Geometry check sheet. Reference: the model listing, model coordinates, mm. Face numbers are marked on the shaded views. A direction names the side the tool comes from. Give positions to 0.01 mm unless a question says otherwise; leave off trailing zeros. Order: outer loops, then holes, each group sorted by start corner. A loop starts at its lowest first (then second) coordinate and runs counter-clockwise, first axis right, second up. Notation, with made-up numbers: M 1.25,31.5 L 58.25,31.5 A19 cw 58.25,61.5 Z; hole C -14.75,49 d1. An arc over 180 degrees is marked long. Answer as CSV lines item,"result". Start each with the question number.
```python
from build123d import *

# Parameters (mm, degrees)
BOSS_EXTRUDE1_DEPTH = 10
BOSS_EXTRUDE2_START = 1
BOSS_EXTRUDE2_DEPTH = 1
SKETCH3_R           = 4
BOSS_EXTRUDE3_DEPTH = 6
SKETCH4_R           = 2
BOSS_EXTRUDE4_DEPTH = 15
FILLET1_R           = 2


with BuildPart() as part:
    # Sketch1 → Boss-Extrude1 (new body)
    with BuildSketch(Plane(origin=(0, 0, 0), x_dir=(1, 0, 0), z_dir=(0, 1, 0))):
        with BuildLine():
            Line((-20.000157194, 1.500878546), (-20.000157194, -1.500878546))
            Line((-20.000157194, -1.500878546), (-0.880639137, -4.921836518))
            ThreePointArc((-0.880639137, -4.921836518), (0, -5), (0.880639137, -4.921836518))
            Line((0.880639137, -4.921836518), (20.000157194, -1.500878546))
            Line((20.000157194, -1.500878546), (20.000157194, 1.500878546))
            Line((20.000157194, 1.500878546), (0.880639137, 4.921836518))
            ThreePointArc((0.880639137, 4.921836518), (0, 5), (-0.880639137, 4.921836518))
            Line((-0.880639137, 4.921836518), (-20.000157194, 1.500878546))
        make_face()
        with BuildLine():
            Line((-19.000157194, -0.663922493), (-19.000157194, 0.663922493))
            Line((-19.000157194, 0.663922493), (-18.824029366, 0.695436148))
            Line((-18.824029366, 0.695436148), (-3.65761322, 3.409085733))
            ThreePointArc((-3.65761322, 3.409085733), (-5, 0), (-3.65761322, -3.409085733))
            Line((-3.65761322, -3.409085733), (-18.824029366, -0.695436148))
            Line((-18.824029366, -0.695436148), (-19.000157194, -0.663922493))
        make_face(mode=Mode.SUBTRACT)
        with BuildLine():
            Line((18.824029366, 0.695436148), (19.000157194, 0.663922493))
            Line((19.000157194, 0.663922493), (19.000157194, -0.663922493))
            Line((19.000157194, -0.663922493), (18.824029366, -0.695436148))
            Line((18.824029366, -0.695436148), (3.65761322, -3.409085733))
            ThreePointArc((3.65761322, -3.409085733), (5, 0), (3.65761322, 3.409085733))
            Line((3.65761322, 3.409085733), (18.824029366, 0.695436148))
        make_face(mode=Mode.SUBTRACT)
    extrude(amount=BOSS_EXTRUDE1_DEPTH)

    # Sketch2 → Boss-Extrude2 (add)
    with BuildSketch(Plane.XZ.offset(BOSS_EXTRUDE2_START)):
        with BuildLine():
            Line((-20.000157194, 1.500878546), (-0.880639137, 4.921836518))
            ThreePointArc((-0.880639137, 4.921836518), (0, 5), (0.880639137, 4.921836518))
            Line((0.880639137, 4.921836518), (20.000157194, 1.500878546))
            Line((20.000157194, 1.500878546), (20.000157194, -1.500878546))
            Line((20.000157194, -1.500878546), (0.880639137, -4.921836518))
            ThreePointArc((0.880639137, -4.921836518), (0, -5), (-0.880639137, -4.921836518))
            Line((-0.880639137, -4.921836518), (-20.000157194, -1.500878546))
            Line((-20.000157194, -1.500878546), (-20.000157194, 1.500878546))
        make_face()
    extrude(amount=-BOSS_EXTRUDE2_DEPTH)

    # Sketch3 → Boss-Extrude3 (add)
    with BuildSketch(Plane(origin=(0, 10, 0), x_dir=(1, 0, 0), z_dir=(0, 1, 0))):
        with Locations(Location((0, 0, 0), (0, 0, 270))):
            Circle(SKETCH3_R)
    extrude(amount=BOSS_EXTRUDE3_DEPTH)

    # Sketch4 → Boss-Extrude4 (add)
    with BuildSketch(Plane(origin=(0, 16, 0), x_dir=(1, 0, 0), z_dir=(0, 1, 0))):
        with Locations(Location((0, 0, 0), (0, 0, 270))):
            Circle(SKETCH4_R)
    extrude(amount=BOSS_EXTRUDE4_DEPTH)

    # Fillet1
    # the kernel refuses this fillet: 2 mm, written as the material it takes off along each edge
    with BuildSketch(Plane(origin=(20.000157194, -5.184780263, 1.500878546), x_dir=(-0.9843673036221247, 0, 0.17612782732920945), z_dir=(0, 1, 0)), Plane(origin=(20.000157194, -5.184780263, -1.500878546), x_dir=(0, 0, 1), z_dir=(0, 1, 0)), Plane(origin=(-20.000157194, 14.184780263, 1.500878546), x_dir=(0.9843673036221245, 0, 0.17612782732920956), z_dir=(0, -1, 0))) as fillet1_piece_1:
        with BuildLine():
            CenterArc((FILLET1_R * 0.836956052521, -FILLET1_R), FILLET1_R, 90, 79.855702636)
            Line((-FILLET1_R * 0.147411251101, -FILLET1_R * 0.823872172671), (0, 0))
            Line((0, 0), (FILLET1_R * 0.836956052521, 0))
        make_face()
    extrude(amount=19.369560525, mode=Mode.SUBTRACT)
    with BuildSketch(Plane(origin=(-20.000157194, -5.184780263, -1.500878546), x_dir=(0, 0, 1), z_dir=(0, 1, 0))) as fillet1_piece_2:
        with BuildLine():
            CenterArc((FILLET1_R * 0.836956052521, FILLET1_R), FILLET1_R, 190.144297364, 79.855702636)
            Line((-FILLET1_R * 0.147411251101, FILLET1_R * 0.823872172671), (0, 0))
            Line((0, 0), (FILLET1_R * 0.836956052521, 0))
        make_face()
    extrude(amount=19.369560525, mode=Mode.SUBTRACT)


solid = part.part
```
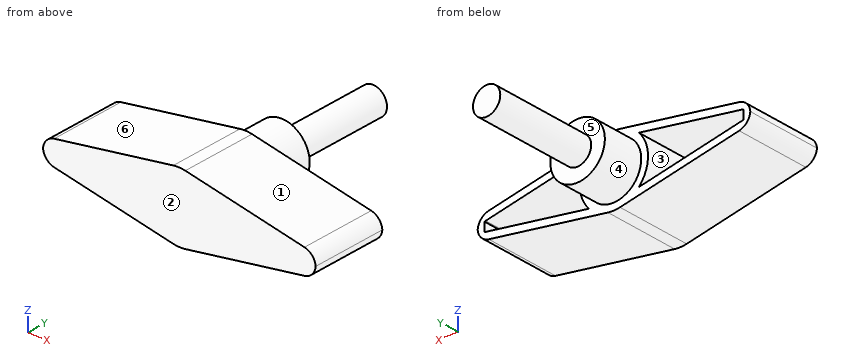
Item 1: Section check D-D on x = -8. Record the boundary of the cut face in (y, z).
Item 2: Draft check along X on the marked faces 1, 2, 3 and 4. Enter one of: pulls with the +X half, pulls with the -X half, needs draft (parallel to the pull), parting line crosses it, or undercut.
Item 3: Access from +Z, -Z, +X, -X, +Y, -Y to the whole of each face (thin tool, end or side, straight path). Record for the marked faces 5 and 6.
Item 4: Depth check by flat-ended pin: pin 1 Ø2 at (x, z) = (10, 0) entering from +Y; pin 2 Ø5.5 at (x, z) = (-11, 1.5) entering from +Y; pin 3 Ø6 at (x, y) = (-4, 3.5) entering from +Z. Enter the tip coordinate at first touch or a pass-through.
Item 5: Section check B-B on y = 18.5. Record the boundary of the cut face in (x, z).
Item 6: Scan lines: line 1 along Y through (x, z) = (3.5, -2.5); line 2 along Z through (x, y) = (-14, 2); line 3 along Y through (x, z) = (6, -1.75). Record each from-to range of solid material in increasing order.
Item 7: Section check C-C on z = -2.5. Record the boundary of the cut face in (x, y), then the cut area to 3 significant figures.
Item 8: Section check A-A on x = 0. Record the boundary of the cut face in (y, z).
Numbers:
1,outline,"M -1,-3.65 L 10,-3.65 L 10,-2.63 L 0,-2.63 L 0,2.63 L 10,2.63 L 10,3.65 L -1,3.65 Z"
2,face 1,"pulls with the +X half"
2,face 2,"needs draft"
2,face 3,"undercut"
2,face 4,"parting line crosses it"
3,face 5,"+Y"
3,face 6,"+Z, -X, +Y, -Y"
4,pin 1,"y = 0"
4,pin 2,"y = 10"
4,pin 3,"z = 4.9"
5,outline,"C 0,0 d4"
6,line 1,"-1 to 10"
6,line 2,"-2.57 to -1.56, 1.56 to 2.57"
6,line 3,"-1 to 0"
7,outline,"M -14.42,-1 L 14.42,-1 L 14.42,10 L 8.74,10 L 8.74,0 L 4.33,0 L 4.33,10 L 3.12,10 L 3.12,16 L -3.12,16 L -3.12,10 L -4.33,10 L -4.33,0 L -8.74,0 L -8.74,10 L -14.42,10 Z"
7,area,"266 mm2"
8,outline,"M -1,-5 L 10,-5 L 10,-4 L 16,-4 L 16,-2 L 31,-2 L 31,2 L 16,2 L 16,4 L 10,4 L 10,5 L -1,5 Z"
